CAD build for the part. Positions are in the model's coordinates, mm. A direction names the side the tool comes from. Give positions to 0.01 mm unless a question says otherwise; leave off trailing zeros. Loops run counter-clockwise (first coordinate to the right, second up) from the corner with the lowest first, then second, coordinate; pieces in that order, holes last. Notation, with made-up numbers: (34.5, 54) -> (51.5, 54) arc R16 cw to (51.5, 80) -> close; hole circle Ø8 at (71, 1.25). An arc over 180 degrees is marked (long way). Use one line per item in the form item = value.
```python
from build123d import *

# Parameters (mm, degrees)
BLOCK_DEPTH                    = 110
SHELL1_T                       = -3
SKETCH2_R                      = 5
CORNER_COLUMNS_DEPTH           = 110
SKETCH3_R                      = 2
FRONT_PANEL_INSERT_HOLES_DEPTH = 7
SKETCH4_R                      = 4.5
PLATE_BOSSES_DEPTH             = 6
SKETCH5_R                      = 2
PLATE_INSERT_HOLES_DEPTH       = 7
SKETCH6_R                      = 8.15
SKETCH6_R_2                    = 6.4
CABLE_GLAND_HOLES_DEPTH        = 4
SKETCH7_W                      = 12
SKETCH7_H                      = 6
CABLE_TIE_BARS_DEPTH           = 12
SKETCH8_W                      = 4
SKETCH8_H                      = 2.5
CABLE_TIE_SLOTS_DEPTH          = 6.02
SKETCH9_W                      = 14
SKETCH9_H                      = 12
USB_ACCESS_DEPTH               = 4
VENTS_LEFT_DEPTH               = 4
VENTS_START                    = -4
VENTS_RIGHT_DEPTH              = 4
SKETCH12_R                     = 4.75
KEYHOLE_HEADS_DEPTH            = 4
KEYHOLE_SLOTS_DEPTH            = 4


with BuildPart() as part:
    # Sketch1 → Block (new body)
    with BuildSketch(Plane.XY):
        with BuildLine():
            Line((-77, 0), (77, 0))
            ThreePointArc((77, 0), (82.656854249, 2.343145751), (85, 8))
            Line((85, 8), (85, 202))
            ThreePointArc((85, 202), (82.656854249, 207.656854249), (77, 210))
            Line((77, 210), (-77, 210))
            ThreePointArc((-77, 210), (-82.656854249, 207.656854249), (-85, 202))
            Line((-85, 202), (-85, 8))
            ThreePointArc((-85, 8), (-82.656854249, 2.343145751), (-77, 0))
        make_face()
    extrude(amount=BLOCK_DEPTH)

    # Shell1
    shell1_openings = [part.faces().sort_by_distance(p)[0] for p in [
        (0, 105, 110),
    ]]
    offset(amount=SHELL1_T, openings=shell1_openings, kind=Kind.INTERSECTION)

    # Sketch2 → Corner columns (add)
    with BuildSketch(Plane.XY):
        with Locations((-78, 7)):
            Circle(SKETCH2_R)
        with Locations((78, 7)):
            Circle(SKETCH2_R)
        with Locations((-78, 203)):
            Circle(SKETCH2_R)
        with Locations((78, 203)):
            Circle(SKETCH2_R)
    extrude(amount=CORNER_COLUMNS_DEPTH)

    # Sketch3 → Front panel insert holes (cut)
    with BuildSketch(Plane.XY.offset(110)):
        with Locations((-78, 7)):
            Circle(SKETCH3_R)
        with Locations((78, 7)):
            Circle(SKETCH3_R)
        with Locations((-78, 203)):
            Circle(SKETCH3_R)
        with Locations((78, 203)):
            Circle(SKETCH3_R)
    extrude(amount=-FRONT_PANEL_INSERT_HOLES_DEPTH, mode=Mode.SUBTRACT)

    # Sketch4 → Plate bosses (add)
    with BuildSketch(Plane.XY.offset(3)):
        with Locations((-65, 46)):
            Circle(SKETCH4_R)
        with Locations((65, 46)):
            Circle(SKETCH4_R)
        with Locations((-65, 190)):
            Circle(SKETCH4_R)
        with Locations((65, 190)):
            Circle(SKETCH4_R)
    extrude(amount=PLATE_BOSSES_DEPTH)

    # Sketch5 → Plate insert holes (cut)
    with BuildSketch(Plane.XY.offset(9)):
        with Locations((-65, 46)):
            Circle(SKETCH5_R)
        with Locations((65, 46)):
            Circle(SKETCH5_R)
        with Locations((-65, 190)):
            Circle(SKETCH5_R)
        with Locations((65, 190)):
            Circle(SKETCH5_R)
    extrude(amount=-PLATE_INSERT_HOLES_DEPTH, mode=Mode.SUBTRACT)

    # Sketch6 → Cable gland holes (cut)
    with BuildSketch(Plane(origin=(0, 0, 0), x_dir=(1, 0, 0), z_dir=(0, 1, 0))):
        with Locations(Location((-50, -45, 0), (0, 0, 270))):
            Circle(SKETCH6_R)
        with Locations(Location((-15, -45, 0), (0, 0, 270))):
            Circle(SKETCH6_R_2)
        with Locations(Location((15, -45, 0), (0, 0, 270))):
            Circle(SKETCH6_R_2)
        with Locations(Location((50, -45, 0), (0, 0, 270))):
            Circle(SKETCH6_R_2)
    extrude(amount=CABLE_GLAND_HOLES_DEPTH, mode=Mode.SUBTRACT)

    # Sketch7 → Cable tie bars (add)
    with BuildSketch(Plane.XY.offset(3)):
        with Locations((-50, 30)):
            Rectangle(SKETCH7_W, SKETCH7_H)
        with Locations((-15, 30)):
            Rectangle(SKETCH7_W, SKETCH7_H)
        with Locations((15, 30)):
            Rectangle(SKETCH7_W, SKETCH7_H)
        with Locations((50, 30)):
            Rectangle(SKETCH7_W, SKETCH7_H)
    extrude(amount=CABLE_TIE_BARS_DEPTH)

    # Sketch8 → Cable tie slots (cut)
    with BuildSketch(Plane(origin=(0, 26.99, 0), x_dir=(1, 0, 0), z_dir=(0, 1, 0))):
        with Locations((-50, -10)):
            Rectangle(SKETCH8_W, SKETCH8_H)
        with Locations((-15, -10)):
            Rectangle(SKETCH8_W, SKETCH8_H)
        with Locations((15, -10)):
            Rectangle(SKETCH8_W, SKETCH8_H)
        with Locations((50, -10)):
            Rectangle(SKETCH8_W, SKETCH8_H)
    extrude(amount=CABLE_TIE_SLOTS_DEPTH, mode=Mode.SUBTRACT)

    # Sketch9 → USB access (cut)
    with BuildSketch(Plane(origin=(-85, 0, 0), x_dir=(0, 0, -1), z_dir=(1, 0, 0))):
        with Locations((-28, 95)):
            Rectangle(SKETCH9_W, SKETCH9_H)
    extrude(amount=USB_ACCESS_DEPTH, mode=Mode.SUBTRACT)

    # Sketch10 → Vents left (cut)
    with BuildSketch(Plane(origin=(-85, 0, 0), x_dir=(0, 0, -1), z_dir=(1, 0, 0))):
        with BuildLine():
            Line((-25, 170.5), (-65, 170.5))
            ThreePointArc((-65, 170.5), (-66.5, 172), (-65, 173.5))
            Line((-65, 173.5), (-25, 173.5))
            ThreePointArc((-25, 173.5), (-23.5, 172), (-25, 170.5))
        make_face()
        with BuildLine():
            Line((-25, 178.5), (-65, 178.5))
            ThreePointArc((-65, 178.5), (-66.5, 180), (-65, 181.5))
            Line((-65, 181.5), (-25, 181.5))
            ThreePointArc((-25, 181.5), (-23.5, 180), (-25, 178.5))
        make_face()
        with BuildLine():
            Line((-25, 186.5), (-65, 186.5))
            ThreePointArc((-65, 186.5), (-66.5, 188), (-65, 189.5))
            Line((-65, 189.5), (-25, 189.5))
            ThreePointArc((-25, 189.5), (-23.5, 188), (-25, 186.5))
        make_face()
    extrude(amount=VENTS_LEFT_DEPTH, mode=Mode.SUBTRACT)

    # Sketch11 → Vents right (cut)
    with BuildSketch(Plane(origin=(85, 0, 0), x_dir=(0, 0, -1), z_dir=(1, 0, 0)).offset(VENTS_START)):
        with BuildLine():
            Line((-25, 170.5), (-65, 170.5))
            ThreePointArc((-65, 170.5), (-66.5, 172), (-65, 173.5))
            Line((-65, 173.5), (-25, 173.5))
            ThreePointArc((-25, 173.5), (-23.5, 172), (-25, 170.5))
        make_face()
        with BuildLine():
            Line((-25, 178.5), (-65, 178.5))
            ThreePointArc((-65, 178.5), (-66.5, 180), (-65, 181.5))
            Line((-65, 181.5), (-25, 181.5))
            ThreePointArc((-25, 181.5), (-23.5, 180), (-25, 178.5))
        make_face()
        with BuildLine():
            Line((-25, 186.5), (-65, 186.5))
            ThreePointArc((-65, 186.5), (-66.5, 188), (-65, 189.5))
            Line((-65, 189.5), (-25, 189.5))
            ThreePointArc((-25, 189.5), (-23.5, 188), (-25, 186.5))
        make_face()
    extrude(amount=VENTS_RIGHT_DEPTH, mode=Mode.SUBTRACT)

    # Sketch12 → Keyhole heads (cut)
    with BuildSketch(Plane.XY):
        with Locations((-45, 165)):
            Circle(SKETCH12_R)
        with Locations((45, 165)):
            Circle(SKETCH12_R)
    extrude(amount=KEYHOLE_HEADS_DEPTH, mode=Mode.SUBTRACT)

    # Sketch13 → Keyhole slots (cut)
    with BuildSketch(Plane.XY):
        with BuildLine():
            Line((-47.15, 165), (-47.15, 176))
            ThreePointArc((-47.15, 176), (-45, 178.15), (-42.85, 176))
            Line((-42.85, 176), (-42.85, 165))
            ThreePointArc((-42.85, 165), (-45, 162.85), (-47.15, 165))
        make_face()
        with BuildLine():
            Line((42.85, 165), (42.85, 176))
            ThreePointArc((42.85, 176), (45, 178.15), (47.15, 176))
            Line((47.15, 176), (47.15, 165))
            ThreePointArc((47.15, 165), (45, 162.85), (42.85, 165))
        make_face()
    extrude(amount=KEYHOLE_SLOTS_DEPTH, mode=Mode.SUBTRACT)


solid = part.part
```
1. Drop flat-ended pins along their axis: P1, Ø2.5, axis at x = -65, y = 190, coming from the +Z side; P2, Ø0.9, axis at x = -83.5, z = 44.5, coming from the -Y side; P3, Ø5, axis at x = -78, y = 7, coming from the +Z side; P4, Ø1.5, axis at x = 83, z = 45, coming from the -Y side. Give the stop position or say it passes through.
Result sheet:
P1 = 2
P2 = 2.77
P3 = 110
P4 = 1.96
2. Cut at C-C, the plane x = 5. Write the cut outline in (y, z), then the cut area to 3 significant figures.
Result sheet:
outline = (0, 0) -> (210, 0) -> (210, 110) -> (207, 110) -> (207, 3) -> (3, 3) -> (3, 110) -> (0, 110) -> close
area = 1,270 mm^2
3. Mould opens along Z. For faces 1 (the flat face through (-44, 30, 9)), 2 (the cylindrical face through (-41.92, 1.48, 43.94)), 3 (the flat face through (66, 44, 9)) say: pulls with the +Z half, pulls with the -Z half, needs draft (parallel to the pull), parting line crosses it, or undercut.
Result sheet:
face_1 = needs draft
face_2 = undercut
face_3 = pulls with the +Z half
4. Cut at A-A, the plane z = 97.5. Write the cut outline in (x, y).
Result sheet:
outline = (-85, 8) arc R8 ccw to (-77, 0) -> (77, 0) arc R8 ccw to (85, 8) -> (85, 202) arc R8 ccw to (77, 210) -> (-77, 210) arc R8 ccw to (-85, 202) -> close; hole (-82, 10) arc R5 cw (long way) to (-75, 3) -> (75, 3) arc R5 cw (long way) to (82, 10) -> (82, 200) arc R5 cw (long way) to (75, 207) -> (-75, 207) arc R5 cw (long way) to (-82, 200) -> close
5. Cut at B-B, the plane z = 45. State how many separate pieces and enclosed holes the cut face has, then the cut area to 3 significant figures.
Result sheet:
separate_pieces = 10
enclosed_holes = 0
area = 2,250 mm^2
6. Tool access for faces 4 (the cylindrical face through (50.281, 1.479, 38.606)), 5 (the flat face through (1, 207, 56)), 6 (the flat face through (-1, 0, 54)): list every direction of +Z, -Z, +X, -X, +Y, -Y with a clear straight run to the whole face (end or side of a thin tool).
Result sheet:
face_4 = -Y
face_5 = +Z
face_6 = +Z, -Z, +X, -X, -Y
7. Drill centre lines: line 1 (X direction, y = 60, z = 102); line 2 (Y direction, x = 78, z = 104.75); line 3 (X direction, y = 1, z = 45). Where is each one in solid material? Low to high.
Result sheet:
line_1 = -85 to -82, 82 to 85
line_2 = 0.06 to 5, 9 to 12, 198 to 201, 205 to 209.94
line_3 = -80.87 to -58.15, -41.85 to -21.4, -8.6 to 8.6, 21.4 to 43.6, 56.4 to 80.87
